Verification items for this drawing (mm, ordinates from the low corner). A direction names the side the tool comes from. Give positions to 0.01 mm unless a question says otherwise; leave off trailing zeros. Order: outer loops, then holes, each group sorted by start corner. A loop starts at its lowest first (then second) coordinate and runs counter-clockwise, first axis right, second up.
(1) Mould release check, pull along Y, two halves, no side actions. Record for the marked faces 1, 2 and 3: pulls with the +Y half, pulls with the -Y half, needs draft (parallel to the pull), parting line crosses it, or undercut.
(2) Sectioned sample at D-D on x = 6. Record the cut outline in (y, z), plus the area to 3 significant figures.
(3) Access from +Z, -Z, +X, -X, +Y, -Y to the whole of each face (thin tool, end or side, straight path). Record for the marked faces 4 and 5.
(4) Sectioned sample at A-A on y = 15. Record the cut outline in (x, z), plus the area to 3 significant figures.
(5) Scan lines: L1, parallel to Y at x = 15, z = 4.7; L2, parallel to Z at x = 27.25, y = 13.25; L3, parallel to Y at x = 15, z = 1.4. Record each from-to range of solid material in increasing order.
(6) Gauge pin test, flat end, axial feed: pin 1 (13 mm diameter, centred on x = 15, y = 15, fed in from +Z). Record the tip position at first contact, or that the pin passes through.
(7) Sectioned sample at C-C on z = 4.9. Record the cut outline in (x, y).
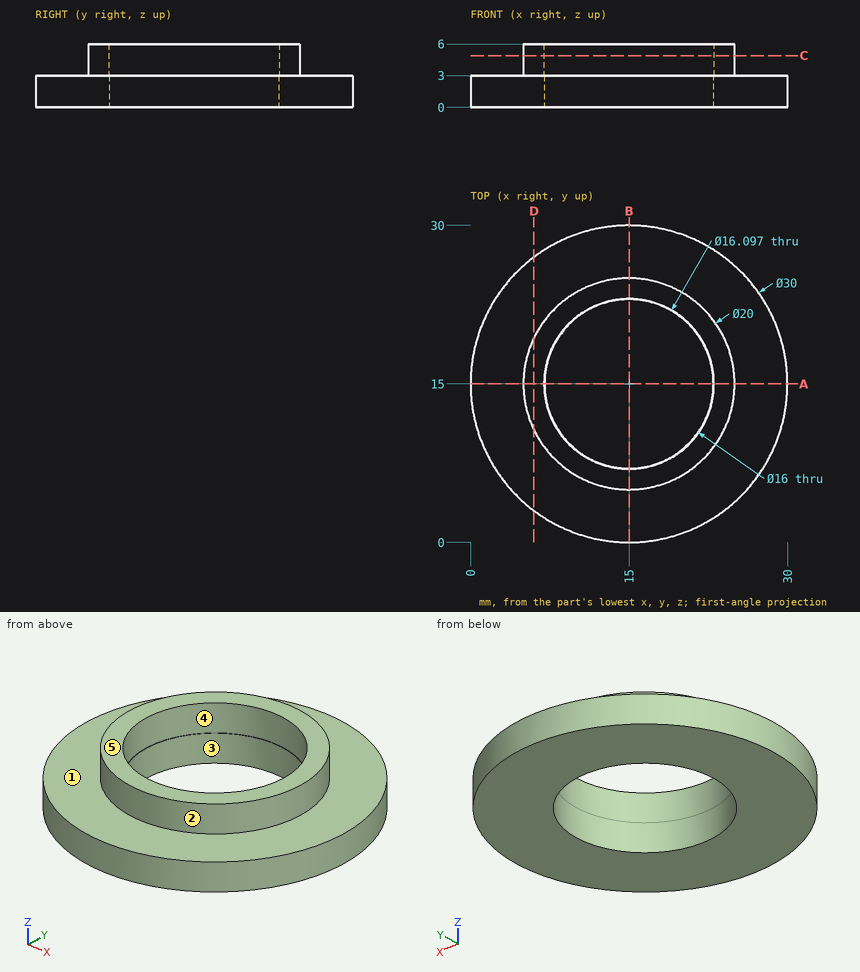
Ans:
1. face 1: needs draft
1. face 2: parting line crosses it
1. face 3: undercut
2. outline: (3, 0) - (27, 0) - (27, 3) - (19.36, 3) - (19.36, 6) - (10.64, 6) - (10.64, 3) - (3, 3) - close
2. area: 98.2 mm2
3. face 4: +Z
3. face 5: +Z, +X, -X, +Y, -Y
4. outline: (0, 0) - (7, 0) - (7, 3) - (6.95, 3) - (6.95, 6) - (5, 6) - (5, 3) - (0, 3) - close; (23, 0) - (30, 0) - (30, 3) - (25, 3) - (25, 6) - (23.05, 6) - (23.05, 3) - (23, 3) - close
4. area: 53.7 mm2
5. L1: y = 5 to 6.95, 23.05 to 25
5. L2: z = 0 to 3
5. L3: y = 0 to 7, 23 to 30
6. pin 1: passes through
7. outline: circle Ø20 at (15, 15); hole circle Ø16.1 at (15, 15)
